Autodesk Inventor part; units mm, degrees
ref_plane "YZ Plane" through (0, 0, 0) normal (1, 0, 0) x (0, 1, 0)
ref_plane "XZ Plane" through (0, 0, 0) normal (0, 1, 0) x (-1, 0, 0)
ref_plane "XY Plane" through (0, 0, 0) normal (0, 0, 1) x (1, 0, 0)
sketch "草图1" plane through (0, 0, 0) normal (0, 0, 1) x (1, 0, 0)
  line L0 (-250, 450) -> (250, 450)
  line L1 (250, 450) -> (250, -450)
  line L2 (250, -450) -> (-250, -450)
  line L3 (-250, -450) -> (-250, 450)
  line L4 (-350, 0) -> (350, 0)
  line L5 (0, -630) -> (0, 630)
  point P0 (0, 0)
  dimension "d0" = 500
  dimension "d1" = 900
extrude "拉伸1" add sketch "草图1" along normal mid plane 700
sketch "草图2" plane through (0, 0, 350) normal (0, 0, 1) x (1, 0, 0)
  line L0 (-225, 425) -> (225, 425)
  line L1 (225, 425) -> (225, -425)
  line L2 (225, -425) -> (-225, -425)
  line L3 (-225, -425) -> (-225, 425)
  line L4 (0, -630) -> (0, 630)
  line L5 (-350, 0) -> (350, 0)
  point P0 (0, 0)
  point P1 (225, 0)
  point P2 (0, -425)
  point P3 (-225, 0)
  point P4 (0, 425)
  dimension "d4" = 850
  dimension "d5" = 450
extrude "拉伸2" cut sketch "草图2" against normal blind 675
sketch "草图3" plane through (0, 0, -325) normal (0, 0, 1) x (1, 0, 0)
  line L0 (225, 425) -> (225, -425)
  line L1 (-225, -425) -> (165, -425)
  line L2 (165, -425) -> (165, -175)
  line L3 (165, -175) -> (-225, -175)
  line L4 (-225, -175) -> (-225, -425)
  point P0 (0, 0)
  point P1 (225, -325)
  dimension "d8" = 250
  dimension "d60" = 390
extrude "拉伸3" cut sketch "草图3" against normal through all
ref_plane "工作平面1" through (180, -425, 350) normal (-1, 0, 0) x (0, 0, 1)
sketch "草图4" plane through (225, -425, 350) normal (-1, 0, 0) x (0, 0, 1)
  line L0 (-400, 280) -> (-310, 280)
  line L1 (-310, 280) -> (-310, 0)
  line L2 (-310, 0) -> (-400, 0)
  line L3 (-400, 0) -> (-400, 280)
  line L4 (-400, -168.792) -> (-400, 811.208)
  line L5 (0, 0) -> (-675, 0)
  line L6 (-700, 875) -> (-700, -25)
  point P0 (-700, 0)
  dimension "d40" = 90
  dimension "d41" = 300
  dimension "d42" = 280
extrude "拉伸4" add sketch "草图4" along normal up to surface (450 mm away)
sketch "草图8" plane through (180, -425, 350) normal (-1, 0, 0) x (0, 0, 1)
  line L0 (-20, 0) -> (-310, 0)
  line L1 (-675, 850) -> (-20, 850)
  line L2 (-20, 850) -> (-20, 0)
  line L3 (-20, 0) -> (-675, 0)
  line L4 (-675, 0) -> (-675, 850)
  line L5 (-675, 850) -> (-675, 0)
  line L6 (0, 850) -> (0, 0)
  point P0 (-350, 425)
  point P1 (-350, 0)
  point P2 (-675, 250)
  point P3 (-275, 0)
  dimension "d33" = 850
  dimension "d117" = 20
extrude "拉伸7" add sketch "草图8" along normal blind 15
sketch "草图12" plane through (225, -425, 40) normal (0, 0, 1) x (1, 0, 0)
  line L0 (0, 280) -> (-45, 280)
  line L1 (-45, 0) -> (0, 0)
  line L2 (-45, 280) -> (0, 280)
  line L3 (0, 280) -> (0, 0)
  line L4 (0, 0) -> (-45, 0)
  line L5 (-45, 0) -> (-45, 280)
  point P0 (-225, 425)
extrude "拉伸8" cut sketch "草图12" against normal up to surface (90 mm away)
sketch "草图6" plane through (225, -145, -50) normal (0, 1, 0) x (1, 0, 0)
  line L0 (-270, -90) -> (-240, -90)
  line L1 (-240, -90) -> (-240, -30)
  line L2 (-240, -30) -> (-270, -30)
  line L3 (-270, -30) -> (-270, -90)
  line L4 (-60, 0) -> (-60, 300)
  line L5 (-450, 0) -> (-450, 300)
  line L6 (-255, 100.8766) -> (-255, -114.3838)
  line L7 (-60, -90) -> (-450, -90)
  line L8 (-60, -90) -> (-450, -90)
  point P0 (0, 0)
  point P1 (-60, 60)
  point P2 (-60, 275)
  point P3 (-450, 60)
  point P4 (-60, -400)
  point P5 (-255, -90)
  dimension "d14" = 60
  dimension "d15" = 30
  dimension "d35" = 390
extrude "拉伸5" cut sketch "草图6" against normal blind 25
sketch "草图7" plane through (225, -170, -50) normal (0, 1, 0) x (1, 0, 0)
  circle A0 centre (-255, -45) radius 6
  circle A1 centre (-255, -65) radius 6
  line L0 (-270.0194, -90) -> (-239.9806, -90)
  line L1 (-60, 0) -> (-60, 300)
  line L2 (-450, 0) -> (-450, 300)
  line L3 (-255, 158.1322) -> (-255, -68.0014)
  line L4 (-240, -90) -> (-270, -90)
  line L5 (-270, -90) -> (-450, -90)
  line L6 (-60, -90) -> (-450, -90)
  line L7 (-60, -90) -> (-240, -90)
  point P0 (-255, -90)
  point P1 (-60, 60)
  point P2 (-60, 275)
  point P3 (-450, 60)
  point P4 (-60, -400)
  point P5 (-255, -90)
  dimension "d9" = 0
  dimension "d20" = 12
  dimension "d21" = 12
  dimension "d22" = 20
  dimension "d23" = 25
  dimension "d38" = 390
extrude "拉伸6" cut sketch "草图7" against normal blind 25
thread "螺纹1"
thread "螺纹2"
fillet "圆角1" radius 10 4 edges at (-250, 450, 0) (250, 450, 0) (-250, -450, 0) (250, -450, 0)
sketch "草图14" plane through (165, -425, -350) normal (-1, 0, 0) x (0, 0, 1)
  line L0 (640, 485) -> (660, 485)
  line L1 (660, 485) -> (660, 405)
  line L2 (660, 405) -> (640, 405)
  line L3 (640, 405) -> (640, 485)
  line L4 (680, 0) -> (680, 850)
  line L5 (680, 0) -> (25, 0)
  point P0 (350, 425)
  point P1 (700, 0)
  point P2 (700, 850)
  dimension "d69" = 80
  dimension "d70" = 20
  dimension "d115" = 20
  dimension "d118" = 405
extrude "拉伸10" cut sketch "草图14" against normal blind 10
sketch "草图15" plane through (175, -425, -350) normal (-1, 0, 0) x (0, 0, 1)
  line L0 (640, 405) -> (640, 485)
  line L1 (660, 405) -> (640, 405)
  line L2 (660, 485) -> (660, 405)
  line L3 (640, 485) -> (660, 485)
  line L4 (640, 405) -> (640, 485)
  line L5 (640, 465) -> (660, 465)
  line L6 (660, 465) -> (660, 425)
  line L7 (660, 425) -> (640, 425)
  line L8 (640, 425) -> (640, 465)
  line L9 (565.3666, 445) -> (668.9353, 445)
  point P0 (350, 425)
  point P1 (640, 445)
  dimension "d74" = 40
extrude "拉伸11" cut sketch "草图15" against normal up to surface (5 mm away) contours L0 L9 L2 L7 | L0 L5 L2 L9
sketch "草图17" plane through (165, -175, -325) normal (-1, 0, 0) x (0, 0, 1)
  line L0 (105, 400) -> (95, 345)
  line L1 (95, 345) -> (575, 225)
  line L2 (575, 225) -> (585, 280)
  line L3 (585, 280) -> (105, 400)
  line L4 (-25, 625) -> (675, 625)
  line L5 (-25, 615) -> (-25, -265)
  point P0 (325, 175)
  dimension "d83" = 480
  dimension "d84" = 55
  dimension "d85" = 225
  dimension "d86" = 130
  dimension "d87" = 120
  dimension "d88" = 120
extrude "拉伸13" cut sketch "草图17" against normal up to surface (15 mm away)
sketch "草图19" plane through (250, -440, 350) normal (1, 0, 0) x (0, 0, -1)
  line L0 (50, 840) -> (130, 840)
  line L1 (130, 840) -> (130, 790)
  line L2 (130, 790) -> (50, 790)
  line L3 (50, 790) -> (50, 840)
  line L4 (700, 890) -> (0, 890)
  line L5 (0, 0) -> (0, 880)
  point P0 (350, 440)
  dimension "d93" = 80
  dimension "d94" = 50
  dimension "d95" = 50
  dimension "d96" = 50
extrude "拉伸15" cut sketch "草图19" against normal blind 10
sketch "草图20" plane through (240, -440, 350) normal (1, 0, 0) x (0, 0, -1)
  line L0 (130, 790) -> (50, 790)
  line L1 (130, 840) -> (130, 790)
  line L2 (50, 840) -> (130, 840)
  line L3 (50, 790) -> (50, 840)
  line L4 (50, 840) -> (130, 840)
  line L5 (75, 840) -> (105, 840)
  line L6 (105, 840) -> (105, 835)
  line L7 (105, 835) -> (75, 835)
  line L8 (75, 835) -> (75, 840)
  line L9 (90, 871.8098) -> (90, 758.1154)
  point P0 (350, 440)
  point P1 (90, 840)
  point P2 (75, 840)
  point P3 (105, 840)
  dimension "d99" = 5
  dimension "d100" = 30
extrude "拉伸16" cut sketch "草图20" against normal up to surface (15 mm away) contours L9 L2 L6 L7 | L7 L8 L2 L9
sketch "草图23" plane through (-225, 425, 350) normal (1, 0, 0) x (0, 0, -1)
  line L0 (100, -375) -> (580, -255)
  line L1 (675, -200) -> (615, -200)
  line L2 (0, -850) -> (0, 0)
  line L3 (0, -850) -> (310, -850)
  line L4 (310, -850) -> (310, -570)
  line L5 (310, -570) -> (400, -570)
  line L6 (400, -570) -> (400, -850)
  line L7 (400, -850) -> (700, -850)
  line L8 (700, -600) -> (700, -850)
  line L9 (675, -600) -> (700, -600)
  line L10 (675, -600) -> (675, 0)
  line L11 (0, 0) -> (675, 0)
  line L12 (615, -200) -> (615, -400)
  line L13 (615, -400) -> (595, -400)
  line L14 (595, -400) -> (595, -165.9896)
  line L15 (595, -165.8218) -> (595, -180)
  line L16 (595, -180) -> (675, -180)
  line L17 (675, -180) -> (675, -200)
  point P0 (350, -425)
  point P1 (650, 0)
  dimension "d110" = 20
  dimension "d111" = 200
  dimension "d112" = 80
extrude "拉伸17" add sketch "草图23" along normal up to surface (390 mm away) contours L1 L12 L13 L14 L16 L10
sketch "草图25" plane through (-250, -440, 350) normal (-1, 0, 0) x (0, 0, 1)
  line L0 (-700, 880) -> (0, 880)
  line L1 (-20, 465) -> (0, 465)
  line L2 (0, 465) -> (0, 365)
  line L3 (0, 365) -> (-20, 365)
  line L4 (-20, 365) -> (-20, 465)
  line L5 (0, 880) -> (0, 0)
  line L6 (0, 0) -> (-700, 0)
  point P0 (-350, 440)
  point P1 (0, 415)
  dimension "d120" = 20
  dimension "d121" = 100
  dimension "d124" = 365
extrude "拉伸19" cut sketch "草图25" against normal through all
properties part number "外壳"
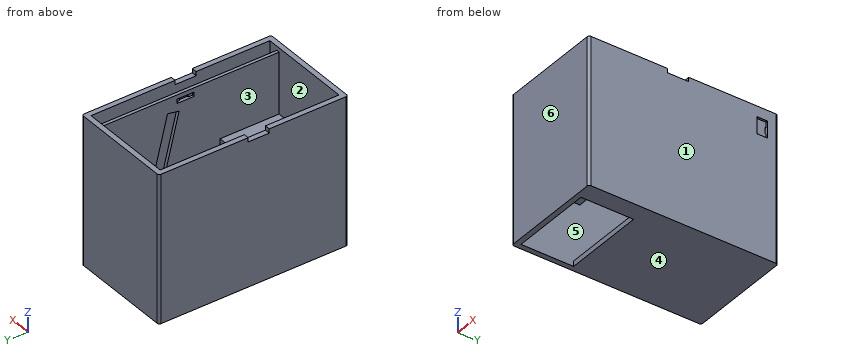
Input: part model. Units: mm. Frame: model coordinates. Face numbers are marked on the shaded views. A direction names the side the tool comes from. Round coordinates to 2 decimals unless told otherwise and drop trailing zeros. Loops run counter-clockwise (first coordinate to the right, second up) from the corner with the lowest first, then second, coordinate; pieces in that order, holes last. Notation, with made-up numbers: M -2.5,72 L 38.5,72 A32 ccw 38.5,98 Z; hole C 51,-1 d10. An arc over 180 degrees is marked long. Answer in a Markdown table with one row per item. Add a question column.
1. Set-up query: the marked faces 1, 2 and 3. Return all of +Z, -Z, +X, -X, +Y, -Y with unobstructed straight access to the full face (end or side cutting, diameter ignored); none if empty.
2. Ray query, probe 1 along X at (y, z) = (-150, 206); probe 2 along Z at (x, y) = (-30, -185); probe 3 along Y at (x, z) = (-213, -264.5). Return the intervals inside material, ascending.
3. Contact query for flat-ended pins moving along their axis: pin 1 (12.5 mm diameter, centred on x = -243, y = -32, fed in from +Z); pin 2 (8 mm diameter, centred on x = -109.5, y = -182.5, fed in from -Z); pin 3 (1.5 mm diameter, centred on x = 49.5, y = 88, fed in from +Z). Output: stop coordinate, or through.
4. Section C-C (z = 158.5). Output: boundary loops of the cut face in (x, y) (3 decimals).
5. Mould query, pull axis Y, two halves, no side actions, for the marked faces 4, 5 and 6. Classes: released by +Y, released by -Y, zero draft, split by the parting line, or undercut.
6. Section A-A (x = 100.5). Output: boundary loops of the cut face in (y, z).
7. Section D-D (y = -267.5). Output: boundary loops of the cut face in (x, z), and give its area (3 significant figures).
8. Section B-B (y = 199.5). Output: boundary loops of the cut face in (x, z), and give its area (3 significant figures).
Values follow:
| question | item | result |
|---|---|---|
| 1 | face 1 | +Z, -Z, +X, +Y, -Y |
| 1 | face 2 | +Z |
| 1 | face 3 | none |
| 2 | probe 1 | -250 to -225, 165 to 180, 225 to 250 |
| 2 | probe 2 | -50 to -11, 1 to 9, 21 to 40 |
| 2 | probe 3 | -450 to -425, 25 to 245, 425 to 450 |
| 3 | pin 1 | z = 330 |
| 3 | pin 2 | z = -50 |
| 3 | pin 3 | z = -245 |
| 4 | outline | M -250,-440 A10 ccw -240,-450 L 240,-450 A10 ccw 250,-440 L 250,440 A10 ccw 240,450 L -240,450 A10 ccw -250,440 Z; hole M -225,-425 L 165,-425 L 165,72.875 L 180,72.875 L 180,-425 L 225,-425 L 225,425 L 180,425 L 180,130.375 L 165,130.375 L 165,425 L -225,425 Z |
| 5 | face 4 | zero draft |
| 5 | face 5 | undercut |
| 5 | face 6 | released by -Y |
| 6 | outline | M -450,-350 L -425,-350 L -425,-50 L -145,-50 L -145,40 L -425,40 L -425,350 L -450,350 Z; M -175,-350 L 450,-350 L 450,350 L 425,350 L 425,-325 L 245,-325 L 245,-245 L 25,-245 L 25,-265 L 225,-265 L 225,-325 L -175,-325 Z |
| 7 | outline | M -250,-350 L -225,-350 L -225,-50 L 165,-50 L 165,-350 L 250,-350 L 250,350 L 225,350 L 225,-325 L 180,-325 L 180,330 L 165,330 L 165,40 L -225,40 L -225,350 L -250,350 Z |
| 7 | area | 81,400 mm^2 |
| 8 | outline | M -250,-350 L 250,-350 L 250,350 L 225,350 L 225,-325 L 180,-325 L 180,-224.64 L 165,-224.64 L 165,-245 L -225,-245 L -225,350 L -250,350 Z; M 165,-118 L 180,-118 L 180,330 L 165,330 Z; hole M -225,-325 L 165,-325 L 165,-265 L -225,-265 Z |
| 8 | area | 62,300 mm^2 |
